Answer from the drawing. Dimensions are ordinates in mm from the lowest x, y and z of the part. A direction names the side the tool comes from. Round coordinates to 2 decimals unless told otherwise and drop trailing zeros. Loops run counter-clockwise (first coordinate to the right, second up) from the corner with the lowest first, then second, coordinate; pieces in that order, holes last. Notation, with made-up numbers: (6, 26) - (43, 26) arc R7 cw to (43, 36) - close; hole circle Ø10 at (-15, 46.5). An arc over 180 degrees is marked (long way). Answer as CSV lines item,"result".
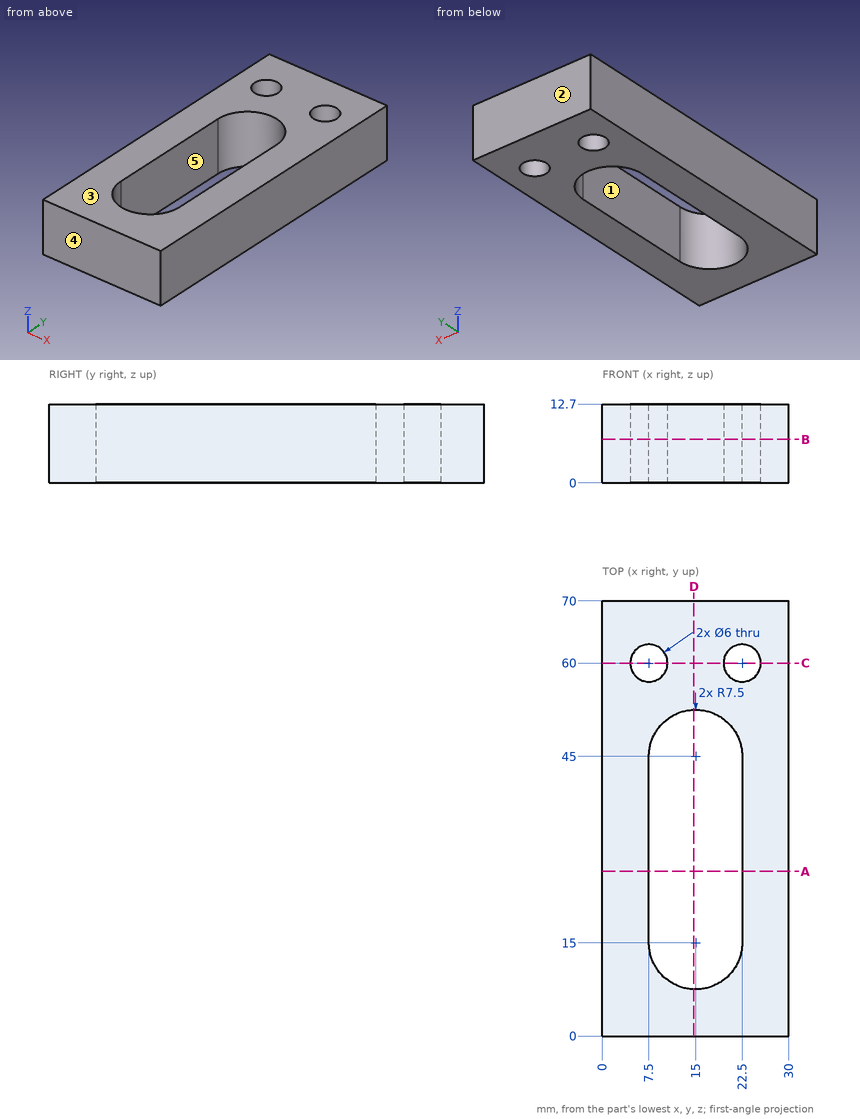
1) Find the intervals of material crossed by line 1 (X direction, y = 30, z = 7.5); line 2 (Y direction, x = 21.75, z = 4); line 3 (X direction, y = 49.5, z = 7.75), in increasing order.
Entries:
line 1,"x = 0 to 7.5, 22.5 to 30"
line 2,"y = 0 to 11.73, 48.27 to 57.1, 62.9 to 70"
line 3,"x = 0 to 9, 21 to 30"
2) A cutting plane is placed at A-A, the plane y = 26.5. Determine the outline of the cut face in (x, z).
Entries:
outline,"(0, 0) - (7.5, 0) - (7.5, 12.7) - (0, 12.7) - close; (22.5, 0) - (30, 0) - (30, 12.7) - (22.5, 12.7) - close"
3) A cutting plane is placed at D-D, the plane x = 14.75. Determine the outline of the cut face in (y, z), plus the area to 3 significant figures.
Entries:
outline,"(0, 0) - (7.5, 0) - (7.5, 12.7) - (0, 12.7) - close; (52.5, 0) - (70, 0) - (70, 12.7) - (52.5, 12.7) - close"
area,"318 mm^2"
4) Each of these flat-tipped pins is pushed along its axis until it touches: P1, Ø1.5, axis at x = 9, y = 27.5, coming from the +Z side; P2, Ø6.5, axis at y = 27.5, z = 6.5, coming from the -X side. Where does it stop, or does it pass through?
Entries:
P1,"passes through"
P2,"stops at x = 0"
5) A tool of negligible diameter and unlimited length cuts with its end or side. For the marked faces 1 and 2, from which of +Z, -Z, +X, -X, +Y, -Y can it reach the whole face along a straight path? Write none if from no direction.
Entries:
face 1,"+Z, -Z"
face 2,"+Z, -Z, +X, -X, +Y"
6) The mould has two halves that part along Y. Classify the marked faces 3, 4 and 5: pulls with the +Y half, pulls with the -Y half, needs draft (parallel to the pull), parting line crosses it, or undercut.
Entries:
face 3,"needs draft"
face 4,"pulls with the -Y half"
face 5,"undercut"
7) A cutting plane is placed at B-B, the plane z = 7. Determine the outline of the cut face in (x, y), plus the area to 3 significant figures.
Entries:
outline,"(0, 0) - (30, 0) - (30, 70) - (0, 70) - close; hole circle Ø6 at (7.5, 60); hole (7.5, 15) arc R7.5 ccw to (22.5, 15) - (22.5, 45) arc R7.5 ccw to (7.5, 45) - close; hole circle Ø6 at (22.5, 60)"
area,"1,420 mm^2"
8) A cutting plane is placed at C-C, the plane y = 60. Determine the outline of the cut face in (x, z).
Entries:
outline,"(0, 0) - (4.5, 0) - (4.5, 12.7) - (0, 12.7) - close; (10.5, 0) - (19.5, 0) - (19.5, 12.7) - (10.5, 12.7) - close; (25.5, 0) - (30, 0) - (30, 12.7) - (25.5, 12.7) - close"
